Autodesk Inventor part; units mm, degrees
ref_plane "YZ Plane" through (0, 0, 0) normal (1, 0, 0) x (0, 1, 0)
ref_plane "XZ Plane" through (0, 0, 0) normal (0, 1, 0) x (-1, 0, 0)
ref_plane "XY Plane" through (0, 0, 0) normal (0, 0, 1) x (1, 0, 0)
sketch "Sketch1" plane through (0, 0, 0) normal (0, 1, 0) x (-1, 0, 0)
  line L0 (67.5, -70) -> (-67.5, -70)
  line L1 (-67.5, -70) -> (-67.5, 70)
  line L2 (-67.5, 70) -> (67.5, 70)
  line L3 (67.5, 70) -> (67.5, -70)
  line L4 (67.5, -70) -> (-67.5, 70) construction
  line L5 (-67.5, -70) -> (67.5, 70) construction
  circle A0 centre (-55.75, -52.5) radius 5.5
  circle A1 centre (55.75, -52.5) radius 5.5
  circle A2 centre (55.75, 47.5) radius 5.5
  circle A3 centre (-55.75, 47.5) radius 5.5
  line L6 (55.75, -52.5) -> (-55.75, -52.5) construction
  line L7 (55.75, 47.5) -> (-55.75, 47.5) construction
  line L8 (0, -70) -> (0, -52.5) construction
  line L9 (0, -52.5) -> (0, 0) construction
  line L10 (0, 0) -> (0, 47.5) construction
  line L11 (0, 70) -> (0, 47.5) construction
  point P0 (0, 0)
  point P1 (0, 0)
  point P2 (0, 0)
  dimension "d0" = 135
  dimension "d1" = 140
  dimension "d2" = 11
  dimension "d4" = 11
  dimension "d5" = 11
  dimension "d6" = 11
  dimension "d7" = 111.5
  dimension "d9" = 100
  dimension "d27" = 22.5
extrude "Extrusion1" add sketch "Sketch1" along normal blind 5
sketch "Sketch3" plane through (0, 5, 0) normal (0, 1, 0) x (1, 0, 0)
  circle A0 centre (55.75, -47.5) radius 5.5 construction
  circle A1 centre (-55.75, -47.5) radius 5.5 construction
  circle A2 centre (-55.75, 52.5) radius 5.5 construction
  circle A3 centre (55.75, 52.5) radius 5.5 construction
  line L0 (67.5, 70) -> (-67.5, 70) construction
  line L1 (-67.5, 70) -> (-67.5, -70) construction
  line L2 (-67.5, -70) -> (67.5, -70) construction
  line L3 (67.5, -70) -> (67.5, 70) construction
  line L4 (-41, -70) -> (41, -70)
  line L5 (-36.7574, -50) -> (36.7574, -50)
  line L6 (-41, -54.2426) -> (-41, -70)
  line L7 (41, -54.2426) -> (41, -70)
  line L8 (-67.5, -70) -> (67.5, -70) construction
  line L9 (-67.5, 70) -> (-67.5, -70) construction
  line L10 (-67.5, 0) -> (67.5, 0) construction
  line L11 (67.5, -70) -> (67.5, 70) construction
  arc A4 (-36.7574, -50) -> (-41, -54.2426) centre (-38.8787, -52.1213) ccw
  line L12 (-41, -50) -> (-38.8787, -52.1213) construction
  line L13 (0, -50) -> (0, -70) construction
  arc A5 (41, -54.2426) -> (36.7574, -50) centre (38.8787, -52.1213) ccw
  line L14 (-41, 70) -> (41, 70)
  line L15 (-36.7574, 50) -> (36.7574, 50)
  line L16 (-41, 54.2426) -> (-41, 70)
  line L17 (41, 54.2426) -> (41, 70)
  arc A6 (-41, 54.2426) -> (-36.7574, 50) centre (-38.8787, 52.1213) ccw
  line L18 (-41, 50) -> (-38.8787, 52.1213) construction
  line L19 (0, 50) -> (0, 70) construction
  arc A7 (36.7574, 50) -> (41, 54.2426) centre (38.8787, 52.1213) ccw
  circle A8 centre (55.75, -47.5) radius 5.5
  circle A9 centre (-55.75, -47.5) radius 5.5
  circle A10 centre (-55.75, 52.5) radius 5.5
  circle A11 centre (55.75, 52.5) radius 5.5
  line L20 (-67.5, 70) -> (67.5, 70)
  line L21 (67.5, 70) -> (67.5, -70)
  line L22 (67.5, -70) -> (-67.5, -70)
  line L23 (-67.5, -70) -> (-67.5, 70)
  point P0 (0, 0)
  point P1 (41, -50)
  point P2 (0, -70)
  point P3 (0, -70)
  point P4 (41, 50)
  point P5 (0, 70)
  point P6 (0, 70)
  dimension "d19" = 82
  dimension "d20" = 20
  dimension "d67" = 6
  dimension "d68" = 45
  dimension "d70" = 73.5147
  dimension "d71" = 15.7574
  dimension "d72" = 120
  dimension "d73" = 26.5
extrude "Extrusion3" cut sketch "Sketch3" against normal blind 1 contours L6 A4 L5 A5 L7 L4 | L14 L17 A7 L15 A6 L16
fillet "Fillet1" radius 2 4 edges at (67.5, 2.5, 70) (-67.5, 2.5, 70) (-67.5, 2.5, -70) (67.5, 2.5, -70)
sketch "Sketch4" plane through (0, 0, 0) normal (0, -1, 0) x (1, 0, 0)
  arc A0 (65.5, -70) -> (67.5, -68) centre (65.5, -68) ccw construction
  line L0 (67.5, -68) -> (67.5, 68) construction
  arc A1 (67.5, 68) -> (65.5, 70) centre (65.5, 68) ccw construction
  line L1 (65.5, 70) -> (-65.5, 70) construction
  arc A2 (-65.5, 70) -> (-67.5, 68) centre (-65.5, 68) ccw construction
  line L2 (-67.5, 68) -> (-67.5, -68) construction
  arc A3 (-67.5, -68) -> (-65.5, -70) centre (-65.5, -68) ccw construction
  line L3 (-65.5, -70) -> (65.5, -70) construction
  circle A4 centre (55.75, 47.5) radius 5.5 construction
  circle A5 centre (-55.75, 47.5) radius 5.5 construction
  circle A6 centre (-55.75, -52.5) radius 5.5 construction
  circle A7 centre (55.75, -52.5) radius 5.5 construction
  line L4 (-41, 70) -> (41, 70)
  line L5 (-41, 65) -> (41, 65)
  line L6 (-41, 70) -> (-41, 65)
  line L7 (41, 70) -> (41, 65)
  line L8 (65.5, 70) -> (-65.5, 70) construction
  point P0 (0, 0)
  point P1 (0, 70)
  point P2 (0, 70)
  point P3 (0, 70)
  dimension "d30" = 82
  dimension "d31" = 5
extrude "Extrusion4" cut sketch "Sketch4" against normal up to next
sketch "Sketch7" plane through (0, 0, 0) normal (0, -1, 0) x (1, 0, 0)
  arc A0 (67.5, 68) -> (65.5, 70) centre (65.5, 68) ccw
  line L0 (67.5, 68) -> (40.95, 68) construction
  line L1 (41, 70) -> (65.5, 70)
  line L2 (40.95, 68) -> (41, 70)
  line L3 (41, 70) -> (32, 70) construction
  line L4 (32, 70) -> (32, 58) construction
  circle A1 centre (32, 58) radius 3
  line L5 (32, 58) -> (-32, 58) construction
  circle A2 centre (-32, 58) radius 3
  line L6 (-67.5, -70) -> (-40.95, -70) construction
  line L7 (-65.5, -70) -> (65.5, -70)
  line L8 (-40.95, -70) -> (-31.95, -70) construction
  line L9 (-31.95, -70) -> (-31.95, -60) construction
  line L10 (-31.95, -60) -> (32.05, -60) construction
  circle A3 centre (-31.95, -60) radius 3
  circle A4 centre (32.05, -60) radius 3
  point P0 (0, 0)
  dimension "d78" = 26.55
  dimension "d79" = 9
  dimension "d80" = 12
  dimension "d81" = 6
  dimension "d82" = 64
  dimension "d84" = 6
  dimension "d85" = 26.55
  dimension "d86" = 9
  dimension "d87" = 10
  dimension "d88" = 64
  dimension "d89" = 6
  dimension "d90" = 6
  dimension "d92" = 63.95
hole "Hole3" at (32, 0, 58) at (-32, 0, 58) at (-31.95, 0, -60) at (32.05, 0, -60) direction (0, 1, 0) diameter 5 end through all countersink diameter 12 countersink angle 90
properties material "Aluminum 6061"
CAD build for the part. Positions are in the model's coordinates, mm. A direction names the side the tool comes from. Round coordinates to 2 decimals unless told otherwise and drop trailing zeros. Write each loop counter-clockwise with the first axis right and the second up, starting at its lowest first coordinate (ties: lowest second). Pieces come first, ordered by that corner, then holes. Notation, with made-up numbers: (22.25, -39.75) -> (29.25, -39.75) arc R23 ccw to (29.25, -8.75) -> close; hole circle Ø8 at (18, 13.25). An arc over 180 degrees is marked (long way). Answer in a Markdown table with one row per item. Add a question column.
Item 1: Saw through at C-C, the plane z = 47.5. Write the cut outline in (x, y).
Item 2: Saw through at B-B, the plane y = 1.95. Count the separate pieces of the cut face and the enclosed holes in it, then the cut area to 3 significant figures.
Item 3: Saw through at A-A, the plane x = 55.75. Write the cut outline in (y, z).
Item 4: Drill centre lines: line 1 (Z direction, x = 32, y = 3.7); line 2 (Z direction, x = 55.75, y = 2.5); line 3 (X direction, y = 3.85, z = 58). Where is each one in solid material? Low to high. Write a range as from..to.
Item 5: Drop flat-ended pins along their axis: pin 1 Ø17.5 at (x, z) = (55.75, 47.5) entering from -Y; pin 2 Ø3 at (x, y) = (4, 2) entering from +Z; pin 3 Ø9 at (x, z) = (-55.75, -52.5) entering from -Y; pin 4 Ø0.5 at (x, y) = (13, 4.5) entering from -Z. Give the stop position or say it passes through.
Item 6: Which spindle directions (+Z, -Z, +X, -X, +Y, -Y) get a long thin tool onto all of the face, cutting with end or side? Do faces 1 (the face through (1, 0, 1)), 2 (the face through (41, 4.5, -50)), 3 (the face through (41, 3, 66)). Say none if no direction does.
Item 7: Saw through at D-D, the plane x = -0.5. Write the cut outline in (y, z).
Item 8: Mould opens along X. For faces 4 (the face through (53, 2, 70)), 5 (the face through (-1, 2, 65)), 6 (the face through (67.5, 2, -1)) say: pulls with the +X half, pulls with the -X half, needs draft (parallel to the pull), parting line crosses it, or undercut.
Findings below:
| question | item | result |
|---|---|---|
| 1 | outline | (-67.5, 0) -> (-61.25, 0) -> (-61.25, 5) -> (-67.5, 5) -> close; (-50.25, 0) -> (50.25, 0) -> (50.25, 5) -> (-50.25, 5) -> close; (61.25, 0) -> (67.5, 0) -> (67.5, 5) -> (61.25, 5) -> close |
| 2 | separate pieces | 1 |
| 2 | enclosed holes | 8 |
| 2 | area | 17,900 mm^2 |
| 3 | outline | (0, -70) -> (5, -70) -> (5, -58) -> (0, -58) -> close; (0, -47) -> (5, -47) -> (5, 42) -> (0, 42) -> close; (0, 53) -> (5, 53) -> (5, 70) -> (0, 70) -> close |
| 4 | line 1 | z = -70..-62.5, -57.5..55.5, 60.5..65 |
| 4 | line 2 | z = -70..-58, -47..42, 53..70 |
| 4 | line 3 | x = -67.5..-34.5, -29.5..29.5, 34.5..67.5 |
| 5 | pin 1 | stops at y = 0 |
| 5 | pin 2 | stops at z = 65 |
| 5 | pin 3 | passes through |
| 5 | pin 4 | stops at z = -50 |
| 6 | face 1 | +Z, -Z, +X, -X, -Y |
| 6 | face 2 | +Y |
| 6 | face 3 | +Z, +Y |
| 7 | outline | (0, -70) -> (4, -70) -> (4, -50) -> (5, -50) -> (5, 50) -> (4, 50) -> (4, 65) -> (0, 65) -> close |
| 8 | face 4 | needs draft |
| 8 | face 5 | undercut |
| 8 | face 6 | pulls with the +X half |
